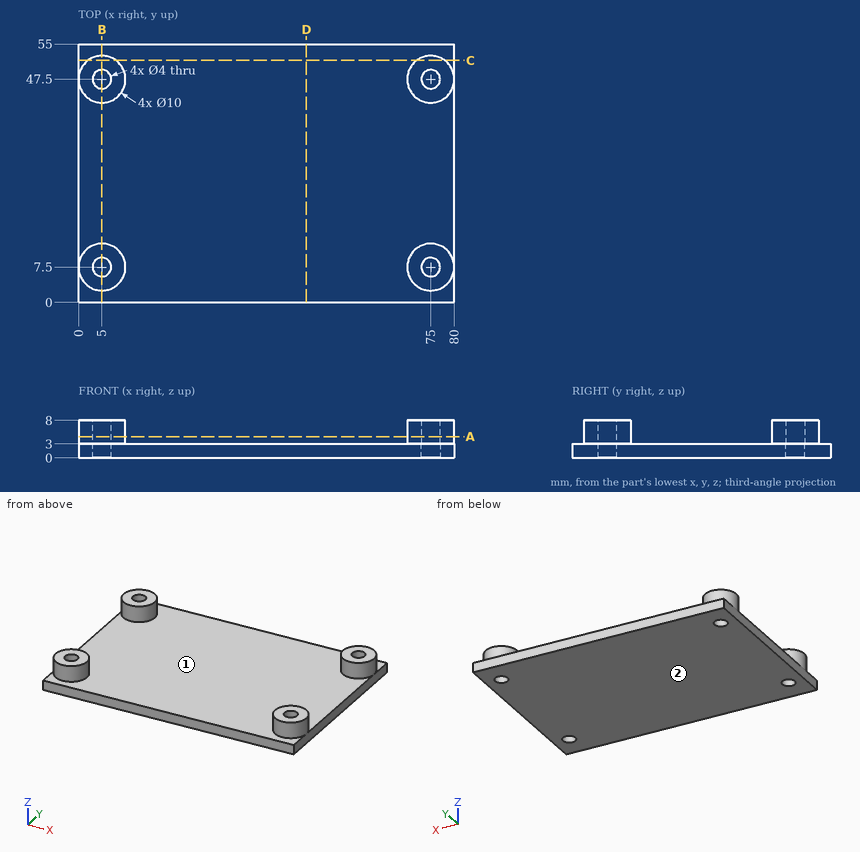
For this review, use the dimensioned drawing (mm, ordinates from the lowest corner) and the shaded views. Round coordinates to 2 decimals unless told otherwise and drop trailing zeros. Order: outer loops, then holes, each group sorted by start corner. A loop starts at its lowest first (then second) coordinate and runs counter-clockwise, first axis right, second up.
1) Draft analysis for pull direction Y (two halves, no side actions). For the marked faces 1 and 2, state which applies: released by +Y, released by -Y, zero draft, split by the parting line, or undercut.
The answers:
face 1: undercut
face 2: zero draft
2) Consider section A-A (z = 4.5). State the section outline as (x, y) points, plus the area to 3 significant figures.
The answers:
outline: circle Ø10 at (5, 7.5); circle Ø10 at (5, 47.5); circle Ø10 at (75, 7.5); circle Ø10 at (75, 47.5); hole circle Ø4 at (5, 7.5); hole circle Ø4 at (5, 47.5); hole circle Ø4 at (75, 7.5); hole circle Ø4 at (75, 47.5)
area: 264 mm2
3) Consider section C-C (y = 51.5). State the section outline as (x, z) points, plus the area to 3 significant figures.
The answers:
outline: (0, 0) - (80, 0) - (80, 3) - (78, 3) - (78, 8) - (72, 8) - (72, 3) - (8, 3) - (8, 8) - (2, 8) - (2, 3) - (0, 3) - close
area: 300 mm2
4) Consider section D-D (x = 48.5). State the section outline as (y, z) points.
The answers:
outline: (0, 0) - (55, 0) - (55, 3) - (0, 3) - close
5) Consider section B-B (x = 5). State the section outline as (y, z) points, plus the area to 3 significant figures.
The answers:
outline: (0, 0) - (5.5, 0) - (5.5, 8) - (2.5, 8) - (2.5, 3) - (0, 3) - close; (9.5, 0) - (45.5, 0) - (45.5, 8) - (42.5, 8) - (42.5, 3) - (12.5, 3) - (12.5, 8) - (9.5, 8) - close; (49.5, 0) - (55, 0) - (55, 3) - (52.5, 3) - (52.5, 8) - (49.5, 8) - close
area: 201 mm2
6) Clearance check with flat-ended pins moving along their axes: pin 1 Ø2.5 at (x, y) = (5, 7.5) entering from +Z; pin 2 Ø5 at (x, y) = (54, 6) entering from +Z. State where each tip first meets the part, or that it passes through.
The answers:
pin 1: passes through
pin 2: stops at z = 3
7) For L1, parallel to Y at x = 75, z = 6.5; L2, parallel to Y at x = 75, z = 1.65; L3, parallel to Y at x = 74, z = 4.75, list the stretches that pass through material, from the lowest coordinate up.
The answers:
L1: y = 2.5 to 5.5, 9.5 to 12.5, 42.5 to 45.5, 49.5 to 52.5
L2: y = 0 to 5.5, 9.5 to 45.5, 49.5 to 55
L3: y = 2.6 to 5.77, 9.23 to 12.4, 42.6 to 45.77, 49.23 to 52.4
